Here's how the part is built. I have some questions about the finished solid (model axes, mm). A direction names the side the tool comes from. Give positions to 0.01 mm unless a question says otherwise; leave off trailing zeros. Loops run counter-clockwise (first coordinate to the right, second up) from the corner with the lowest first, then second, coordinate; pieces in that order, holes last. Notation, with made-up numbers: (68.5, 27.25) - (119.5, 27.25) arc R19 cw to (119.5, 35.25) - close; hole circle Ø3 at (16.25, 71.25). An arc over 180 degrees is marked (long way). Use a Markdown table: item, result.
from build123d import *

# Parameters (mm, degrees)
F0_W     = 2
F0_H     = 48
F1_DEPTH = 16
F2_DEPTH = 2
F4_D     = 4
F6_D     = 4


with BuildPart() as f1:
    # F0 (on Front) → F1 (new body)
    with BuildSketch(Plane.XZ):
        with Locations((-6.5, 0)):
            Rectangle(F0_W, F0_H)
    extrude(amount=F1_DEPTH)

    # F0 (on Front) → F2 (join)
    with BuildSketch(Plane.XZ):
        with Locations((-6.5, 0)):
            Rectangle(F0_W, F0_H)
        with BuildLine():
            Line((-5.5, 24), (-5.5, -24))
            Line((-5.5, -24), (2.5, -24))
            ThreePointArc((2.5, -24), (6.035534, -22.535534), (7.5, -19))
            Line((7.5, -19), (7.5, -12))
            Line((7.5, -12), (7.5, 12))
            Line((7.5, 12), (7.5, 19))
            ThreePointArc((7.5, 19), (6.035534, 22.535534), (2.5, 24))
            Line((2.5, 24), (-5.5, 24))
        make_face()
        with BuildLine():
            Line((7.5, 12), (7.5, -12))
            ThreePointArc((7.5, -12), (19.5, 0), (7.5, 12))
        make_face()
    extrude(amount=F2_DEPTH)

    # F4 (through all)
    with Locations(Plane.XZ.offset(2)):
        with Locations((7.5, 0)):
            Hole(F4_D / 2)

    # F6 (through all)
    with Locations(Plane.YZ.offset(-5.5)):
        with Locations((-9, -12.428912), (-9, 11.571088)):
            Hole(F6_D / 2)


solid = f1.part
(1) Suppose I cut it at D-D on z = 17. Write out the boundary of the cut face in (x, y).
A:
| item | result |
|---|---|
| outline | (-7.5, -16) - (-5.5, -16) - (-5.5, -2) - (7.5, -2) - (7.5, 0) - (-7.5, 0) - close |
(2) Suppose I cut it at A-A on z = 0. Write out the boundary of the cut face in (x, y), plus the area to 3 significant figures.
A:
| item | result |
|---|---|
| outline | (-7.5, -16) - (-5.5, -16) - (-5.5, -2) - (5.5, -2) - (5.5, 0) - (-7.5, 0) - close; (9.5, -2) - (19.5, -2) - (19.5, 0) - (9.5, 0) - close |
| area | 74.0 mm2 |
(3) Will these pins go through, and if not, where does the flat tip stop? pin 1 (4 mm diameter, centred on y = -3, z = -11.5, fed in from +X); pin 2 (6 mm diameter, centred on x = -0.5, z = 18, fed in from +Y); pin 3 (1 mm diameter, centred on y = -14, z = -6, fed in from +X); pin 4 (3 mm diameter, centred on y = -9, z = 11.57, fed in from -X).
A:
| item | result |
|---|---|
| pin 1 | x = 14.47 |
| pin 2 | y = 0 |
| pin 3 | x = -5.5 |
| pin 4 | through |
(4) Suppose I cut it at B-B on y = -9. Write out the boundary of the cut face in (x, z), plus the area to 3 significant figures.
A:
| item | result |
|---|---|
| outline | (-7.5, -24) - (-5.5, -24) - (-5.5, -14.43) - (-7.5, -14.43) - close; (-7.5, -10.43) - (-5.5, -10.43) - (-5.5, 9.57) - (-7.5, 9.57) - close; (-7.5, 13.57) - (-5.5, 13.57) - (-5.5, 24) - (-7.5, 24) - close |
| area | 80.0 mm2 |
(5) Suppose I cut it at C-C on x = 8.5. Write out the boundary of the cut face in (y, z).
A:
| item | result |
|---|---|
| outline | (-2, -11.96) - (0, -11.96) - (0, -1.73) - (-2, -1.73) - close; (-2, 1.73) - (0, 1.73) - (0, 11.96) - (-2, 11.96) - close |
(6) We'd pull the mould along Z, two halves only. Please class faces 1 (the face through (-6.514, -8.74, 13.554)), 2 (the face through (-6, -6, -24)), 3 (the face through (4, -2, 0)): pulls with the +Z half, pulls with the -Z half, needs draft (parallel to the pull), parting line crosses it, or undercut.
A:
| item | result |
|---|---|
| face 1 | undercut |
| face 2 | pulls with the -Z half |
| face 3 | needs draft |
(7) On a 3-axis mill with a long thin cutter (end or side, diameter ignored), from which of +Z, -Z, +X, -X, +Y, -Y can I reach the whole of each face in a straight line? I mean faces 4 (the face through (-5.5, -9, 0)), 5 (the face through (7.5, -1, 15)), 6 (the face through (7.5, -1, -16)). Say none if no direction works.
A:
| item | result |
|---|---|
| face 4 | +Z, -Z, +X, -Y |
| face 5 | +Z, +X, +Y, -Y |
| face 6 | -Z, +X, +Y, -Y |
(8) If I drill on line 1 (Z direction, x = -7, y = -9); line 2 (X direction, y = -8.75, z = -2.5); line 3 (X direction, y = -1, z = 1), over which ranges is the centre line in solid material (lowest first)?
A:
| item | result |
|---|---|
| line 1 | -24 to -14.43, -10.43 to 9.57, 13.57 to 24 |
| line 2 | -7.5 to -5.5 |
| line 3 | -7.5 to 5.77, 9.23 to 19.46 |
